Geometry check sheet. Reference: the model listing, model coordinates, mm. Face numbers are marked on the shaded views. A direction names the side the tool comes from. Give positions to 0.01 mm unless a question says otherwise; leave off trailing zeros. Order: outer loops, then holes, each group sorted by start corner. A loop starts at its lowest first (then second) coordinate and runs counter-clockwise, first axis right, second up. Notation, with made-up numbers: M 41,-30 L 96,-30 A21 ccw 96,-19 Z; hole C -2,14 d10. An arc over 180 degrees is marked long. Use CSV: the item, a comma, the result in double quotes. Start each with the question number.
from build123d import *

# Parameters (mm, degrees)
AUFSATZ_LINEAR_AUSTRAGEN1_DEPTH                      = 6.74
AUFSATZ_LINEAR_AUSTRAGEN1_DEPTH_BACK                 = 3.42
SKIZZE1_R                                            = 1.385
SCHNITT_LINEAR_AUSTRAGEN1_DEPTH                      = 24.827593248
SCHNITT_LINEAR_AUSTRAGEN1_DEPTH_BACK                 = 24.827593248
SKIZZE2_W                                            = 16.035180953
SKIZZE2_H                                            = 1.68
SKIZZE3_R                                            = 1.2
SCHNITT_LINEAR_AUSTRAGEN2_DEPTH                      = 2.16
SKIZZE4_R                                            = 0.35
AUFSATZ_LINEAR_AUSTRAGEN2_DEPTH                      = 7
LINEAR_AUSTRAGEN_D_NN1_DEPTH                         = 0.55
FORMSENKUNG_F_R_M3_SENKSCHRAUBE_MIT_SCHL_D           = 3
FORMSENKUNG_F_R_M3_SENKSCHRAUBE_MIT_SCHL_DEPTH       = 11
FORMSENKUNG_F_R_M3_SENKSCHRAUBE_MIT_SCHL_CSINK_D     = 5.6
FORMSENKUNG_F_R_M3_SENKSCHRAUBE_MIT_SCHL_CSINK_ANGLE = 90
FORMSENKUNG_F_R_M3_SENKSCHRAUBE_MIT_SCHL_TIP         = 0.901290929


with BuildPart() as part:
    # Skizze1 → Aufsatz-Linear austragen1 (new, two sides: drawn at the far end of the back side and taken through both)
    with BuildSketch(Plane(origin=(0, 0, 0), x_dir=(1, 0, 0), z_dir=(0, 1, 0)).offset(-AUFSATZ_LINEAR_AUSTRAGEN1_DEPTH_BACK)):
        Polygon((-13.21, -18.65), (-13.21, -12.79), (-7.6, -7.09), (7.6, -7.09), (13.21, -12.79), (13.21, -18.65), align=None)
        with Locations(Location((-10.48, -15.75, 0), (0, 0, 270))):
            Circle(SKIZZE1_R, mode=Mode.SUBTRACT)
        with Locations(Location((10.48, -15.75, 0), (0, 0, 90))):
            Circle(SKIZZE1_R, mode=Mode.SUBTRACT)
    extrude(amount=AUFSATZ_LINEAR_AUSTRAGEN1_DEPTH + AUFSATZ_LINEAR_AUSTRAGEN1_DEPTH_BACK)

    # Skizze2 → Schnitt-Linear austragen1 (cut, two sides: drawn at the far end of the back side and taken through both)
    with BuildSketch(Plane(origin=(0, 0, 0), x_dir=(0, 0, -1), z_dir=(1, 0, 0)).offset(-SCHNITT_LINEAR_AUSTRAGEN1_DEPTH_BACK)):
        with Locations((-5.332409524, 0.44)):
            Rectangle(SKIZZE2_W, SKIZZE2_H)
    extrude(amount=SCHNITT_LINEAR_AUSTRAGEN1_DEPTH + SCHNITT_LINEAR_AUSTRAGEN1_DEPTH_BACK, mode=Mode.SUBTRACT)

    # Skizze3 → Schnitt-Linear austragen2 (cut)
    with BuildSketch(Plane(origin=(0, 6.74, 0), x_dir=(1, 0, 0), z_dir=(0, 1, 0))):
        with Locations(Location((6.35, -15.75, 0), (0, 0, 270))):
            Circle(SKIZZE3_R)
        with Locations(Location((-6.35, -15.75, 0), (0, 0, 90))):
            Circle(SKIZZE3_R)
    extrude(amount=-SCHNITT_LINEAR_AUSTRAGEN2_DEPTH, mode=Mode.SUBTRACT)

    # Skizze4 → Aufsatz-Linear austragen2 (add)
    with BuildSketch(Plane.XY.offset(18.65)):
        with Locations((0, -1.9)):
            Circle(SKIZZE4_R)
        with Locations((2.54, -1.9)):
            Circle(SKIZZE4_R)
        with Locations((5.08, -1.9)):
            Circle(SKIZZE4_R)
        with Locations(Location((-2.54, -1.9, 0), (0, 0, 180))):
            Circle(SKIZZE4_R)
        with Locations(Location((-5.08, -1.9, 0), (0, 0, 180))):
            Circle(SKIZZE4_R)
    extrude(amount=AUFSATZ_LINEAR_AUSTRAGEN2_DEPTH)

    # Skizze5 → Linear-Austragen-D_nn1 (add, symmetric)
    with BuildSketch(Plane(origin=(8.1, 0, 0), x_dir=(0, 0, -1), z_dir=(1, 0, 0))):
        with BuildLine():
            Line((-18.65, -1.57), (-22.05, -1.57))
            ThreePointArc((-22.05, -1.57), (-22.509619408, -1.379619408), (-22.7, -0.92))
            Line((-22.7, -0.92), (-22.7, 3.58))
            ThreePointArc((-22.7, 3.58), (-22.509619408, 4.039619408), (-22.05, 4.23))
            Line((-22.05, 4.23), (-18.65, 4.23))
            Line((-18.65, 4.23), (-18.65, 4.93))
            Line((-18.65, 4.93), (-22.05, 4.93))
            ThreePointArc((-22.05, 4.93), (-23.004594155, 4.534594155), (-23.4, 3.58))
            Line((-23.4, 3.58), (-23.4, -0.92))
            ThreePointArc((-23.4, -0.92), (-23.004594155, -1.874594155), (-22.05, -2.27))
            Line((-22.05, -2.27), (-18.65, -2.27))
            Line((-18.65, -2.27), (-18.65, -1.57))
        make_face()
    linear_austragen_d_nn1 = extrude(amount=LINEAR_AUSTRAGEN_D_NN1_DEPTH, both=True)

    # Spiegeln1: Linear-Austragen-D_nn1 across plane
    add(linear_austragen_d_nn1.mirror(Plane(origin=(0, 0, 0), x_dir=(0, 0, 1), z_dir=(1, 0, 0))))

    # Formsenkung f_r M3 Senkschraube mit Schl
    with Locations(Plane(origin=(0, -3.42, 0), x_dir=(-1, 0, 0), z_dir=(0, -1, 0))):
        with Locations((-10.48, -15.75), (10.48, -15.75)):
            CounterSinkHole(FORMSENKUNG_F_R_M3_SENKSCHRAUBE_MIT_SCHL_D / 2, FORMSENKUNG_F_R_M3_SENKSCHRAUBE_MIT_SCHL_CSINK_D / 2, depth=FORMSENKUNG_F_R_M3_SENKSCHRAUBE_MIT_SCHL_DEPTH, counter_sink_angle=FORMSENKUNG_F_R_M3_SENKSCHRAUBE_MIT_SCHL_CSINK_ANGLE)
            with Locations((0, 0, -(FORMSENKUNG_F_R_M3_SENKSCHRAUBE_MIT_SCHL_DEPTH + FORMSENKUNG_F_R_M3_SENKSCHRAUBE_MIT_SCHL_TIP / 2))):  # 118° drill point
                Cone(0, FORMSENKUNG_F_R_M3_SENKSCHRAUBE_MIT_SCHL_D / 2, FORMSENKUNG_F_R_M3_SENKSCHRAUBE_MIT_SCHL_TIP, mode=Mode.SUBTRACT)


solid = part.part
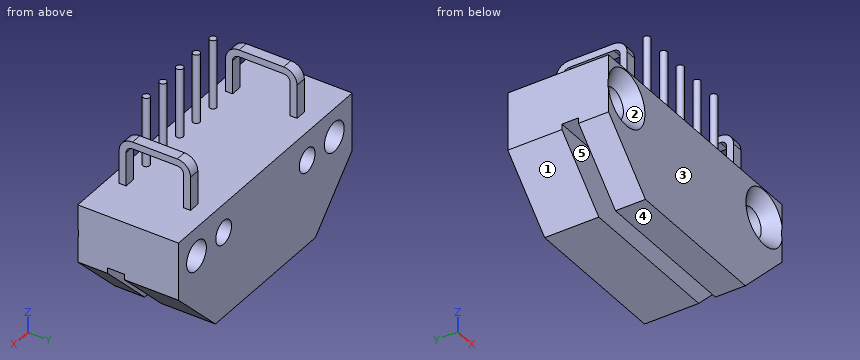
(1) Go/stop test with flat-tipped pins: P1, Ø4, axis at x = 8, y = -1, coming from the +Z side; P2, Ø3, axis at x = 0, y = 1, coming from the +Z side; P3, Ø2, axis at x = 6.35, z = 15.75, coming from the +Y side. Record where each tip stops, or that it passes through.
(2) Thickness scan on line 1 (X direction, y = 1.5, z = 15.75); line 2 (X direction, y = 5.1, z = 15.75); line 3 (Y direction, x = -0.75, z = 9.5). Record the ranges inside material, lowest first.
(3) Sectioned sample at C-C on x = 3.75. Record the cut outline in (y, z).
(4) Draft check along Z on the marked faces 1, 2 and 3. Enter one of: +Z half, -Z half, draft (parallel to the pull), parting line (faces both ways), or undercut.
(5) Sectioned sample at D-D on z = 15.75. Record the cut outline in (x, y), then the cut area to 3 significant figures.
(6) Sectioned sample at A-A on y = 3. Record the cut outline in (x, z), then the cut area to 3 significant figures.
(7) Sectioned sample at B-B on z = 21. Give the number of separate pieces and of enclosed holes in the cut face, then the cut area to 3 significant figures.
(8) Access from +Z, -Z, +X, -X, +Y, -Y to the whole of each face (thin tool, end or side, straight path). Record for the marked faces 4 and 5.
Responses:
1,P1,"z = 23.4"
1,P2,"z = 18.65"
1,P3,"y = 4.58"
2,line 1,"-13.21 to -11.98, -8.98 to 8.98, 11.98 to 13.21"
2,line 2,"-13.21 to -11.98, -8.98 to -7.55, -5.15 to 5.15, 7.55 to 8.98, 11.98 to 13.21"
2,line 3,"-3.42 to -0.4, 1.28 to 6.74"
3,outline,"M -3.42,7.09 L -0.4,7.09 L -0.4,13.35 L 1.28,13.35 L 1.28,7.09 L 6.74,7.09 L 6.74,18.65 L -3.42,18.65 Z"
4,face 1,"-Z half"
4,face 2,"undercut"
4,face 3,"draft"
5,outline,"M -13.21,-3.35 L -11.98,-2.12 L -11.98,6.74 L -13.21,6.74 Z; M -8.98,-2.12 L -7.68,-3.42 L 7.68,-3.42 L 8.98,-2.12 L 8.98,6.74 L 7.55,6.74 L 7.55,4.58 L 5.15,4.58 L 5.15,6.74 L -5.15,6.74 L -5.15,4.58 L -7.55,4.58 L -7.55,6.74 L -8.98,6.74 Z; M 11.98,-2.12 L 13.21,-3.35 L 13.21,6.74 L 11.98,6.74 Z"
5,area,"194 mm2"
6,outline,"M -13.21,12.79 L -7.6,7.09 L 7.6,7.09 L 13.21,12.79 L 13.21,18.65 L -13.21,18.65 Z; M -8.65,22.7 L -7.55,22.7 L -7.55,23.4 L -8.65,23.4 Z; M 7.55,22.7 L 8.65,22.7 L 8.65,23.4 L 7.55,23.4 Z; hole C -10.48,15.75 d3; hole C 10.48,15.75 d3"
6,area,"261 mm2"
7,separate pieces,"9"
7,enclosed holes,"0"
7,area,"5.00 mm2"
8,face 4,"-Z, +X, -X, +Y, -Y"
8,face 5,"-Z, +X, -X"
